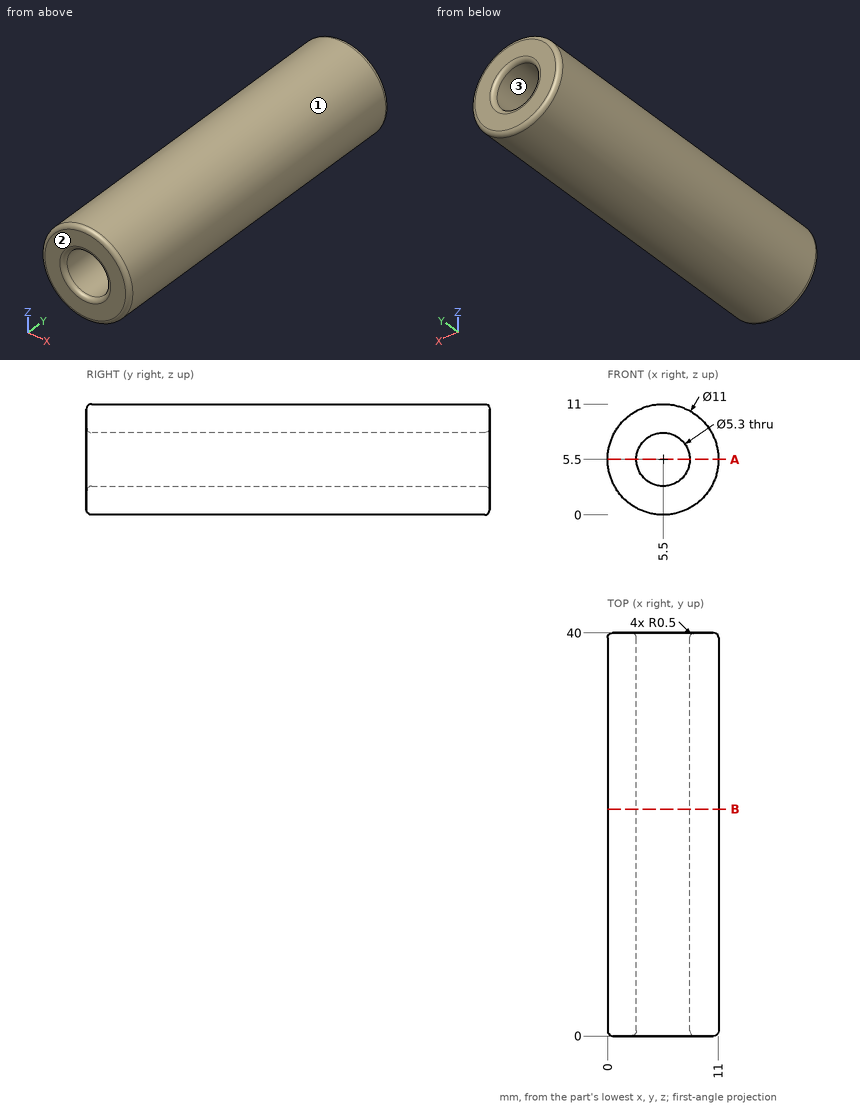
Geometry: see drawing. Coordinates: mm, zero at the bounding-box minimum. Coordinates: 2 decimals unless noted, no trailing zeros. Write each loop counter-clockwise with the first axis right and the second up, starting at its lowest first coordinate (ties: lowest second). Pieces come first, ordered by that corner, then holes. Notation, with made-up numbers: M -25.5,-32.75 L 14.5,-32.75 A18 ccw 14.5,-6.75 Z; hole C 88.25,-15.75 d10. An arc over 180 degrees is marked long. Use CSV: the item, a comma, the result in double quotes. Start each with the question number.
1. First-contact query: P1, Ø3, axis at y = 35.5, z = 4.5, coming from the -X side; P2, Ø3, axis at x = 5.5, z = 5.5, coming from the +Y side. Flat tips, straight axial feed; report the tip coordinate or a pass-through.
2. Mould query, pull axis Z, two halves, no side actions, for the marked faces 1, 2 and 3. Classes: pulls with the +Z half, pulls with the -Z half, needs draft (parallel to the pull), parting line crosses it, or undercut.
3. Cut plane B-B on y = 22.5. Return the cut outline in (x, z).
4. Cut plane A-A on z = 5.5. Return the cut outline in (x, y).
5. Ray query, probe 1 along X at (y, z) = (16, 5.5); probe 2 along X at (y, z) = (4, 4.75). Return the intervals inside material, ascending.
Entries:
1,P1,"x = 0"
1,P2,"through"
2,face 1,"parting line crosses it"
2,face 2,"needs draft"
2,face 3,"undercut"
3,outline,"C 5.5,5.5 d11; hole C 5.5,5.5 d5.3"
4,outline,"M 0,0.5 A0.5 ccw 0.5,0 L 2.35,0 A0.5 ccw 2.85,0.5 L 2.85,39.5 A0.5 ccw 2.35,40 L 0.5,40 A0.5 ccw 0,39.5 Z; M 8.15,0.5 A0.5 ccw 8.65,0 L 10.5,0 A0.5 ccw 11,0.5 L 11,39.5 A0.5 ccw 10.5,40 L 8.65,40 A0.5 ccw 8.15,39.5 Z"
5,probe 1,"0 to 2.85, 8.15 to 11"
5,probe 2,"0.05 to 2.96, 8.04 to 10.95"
